The listing builds one solid part. Answer for the finished solid, in the listing's coordinates (mm). Face numbers are marked on the shaded views. A direction names the side the tool comes from. Round coordinates to 2 decimals unless told otherwise and drop trailing zeros. Loops run counter-clockwise (first coordinate to the right, second up) from the corner with the lowest first, then second, coordinate; pieces in that order, holes last. Notation, with made-up numbers: (-36, -11.5) - (-19, -11.5) arc R17 cw to (-19, 5.5) - close; hole circle Ø5 at (79.5, -12.75). An arc over 180 degrees is marked (long way). Write item = value, one per line. Start each with the question number.
1) Section A-A, the plane y = -25.5 is taken. Determine the outline of the cut face in (x, z), and give its area (3 significant figures).
2) Straight lines are drawn through the part: line 1 along Y through (x, z) = (55, 8.75); line 2 along X through (y, z) = (-25, 6); line 3 along X through (y, z) = (-6, 7.5). For each, find the intervals that lie inside material, in ascending order.
3) Section C-C, the plane x = 55 is taken. Determine the outline of the cut face in (y, z).
4) Section B-B, the plane z = 8.75 is taken. Determine the outline of the cut face in (x, y).
5) Section D-D, the plane z = 3.25 is taken. Determine the outline of the cut face in (x, y).
6) For a pull along X with two mould halves and no side action, classify the marked faces 1, 2 and 3 as released by +X, released by -X, zero draft, split by the parting line, or undercut.
7) A tool of negligible diameter and unlimited length cuts with its end or side. For the marked faces 4, 5, 6, 7 and 8, from which of +Z, -Z, +X, -X, +Y, -Y can it reach the whole face along a straight path? Write none if from no direction.
8) Given pin 1 Ø5 at (y, z) = (-31.5, 6.5) entering from -X; pin 2 Ø1.5 at (x, y) = (47.5, -11.5) entering from +Z; pin 3 Ø1.5 at (y, z) = (-21, 2.5) entering from +X; pin 4 Ø4 at (y, z) = (-24, 8.5) entering from +X, each flat-ended and moving along its own axis, determine where each tip first touches the part or whether it passes through.
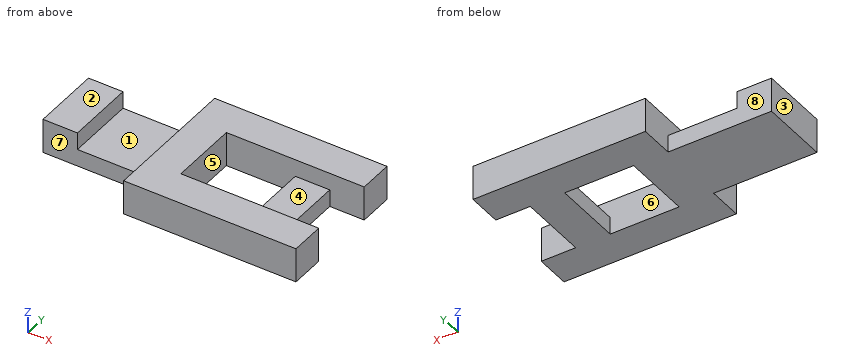
from build123d import *

# Parameters (mm, degrees)
F1_DEPTH  = 40
F3_DEPTH  = 10
F5_DEPTH  = 10
F6_W      = 10
F6_H      = 20
F7_DEPTH  = 25
F6_W_2    = 30
F8_DEPTH  = 5
F9_W      = 20
F9_H      = 20
F10_DEPTH = 25
F11_DEPTH = 10


with BuildPart() as f1:
    # F0 (on Front) → F1 (new body)
    with BuildSketch(Plane.XZ):
        Polygon((0, 10), (0, 0), (80, 0), (80, 10), (40, 10), (40, 5), (10, 5), (10, 10), align=None)
    extrude(amount=F1_DEPTH)

    # F2 (on face) → F3 (cut)
    with BuildSketch(Plane.XZ.offset(40)):
        Polygon((10, 10), (0, 10), (0, 0), (40, 0), (40, 5), (10, 5), align=None)
    extrude(amount=-F3_DEPTH, mode=Mode.SUBTRACT)

    # F4 (on face) → F5 (cut)
    with BuildSketch(Plane(origin=(0, 0, 0), x_dir=(-1, 0, 0), z_dir=(0, 1, 0))):
        Polygon((-40, 0), (0, 0), (0, 10), (-10, 10), (-10, 5), (-40, 5), align=None)
    extrude(amount=-F5_DEPTH, mode=Mode.SUBTRACT)

    # F6 (on face) → F7 (cut)
    with BuildSketch(Plane.XY.offset(10)):
        with Locations((75, -20)):
            Rectangle(F6_W, F6_H)
    extrude(amount=-F7_DEPTH, mode=Mode.SUBTRACT)

    # F6 (on face) → F8 (cut)
    with BuildSketch(Plane.XY.offset(10)):
        with Locations((55, -20)):
            Rectangle(F6_W_2, F6_H)
    extrude(amount=-F8_DEPTH, mode=Mode.SUBTRACT)

    # F9 (on face) → F10 (cut)
    with BuildSketch(Plane.XY.offset(10)):
        with Locations((50, -20)):
            Rectangle(F9_W, F9_H)
    extrude(amount=-F10_DEPTH, mode=Mode.SUBTRACT)

    # F9 (on face) → F11 (join)
    with BuildSketch(Plane.XY.offset(10)):
        Polygon((30, -40), (40, -40), (40, -30), (40, -10), (40, 0), (30, 0), align=None)
    extrude(amount=-F11_DEPTH)


solid = f1.part
Geometry check:
q1.outline = (0, 0) - (40, 0) - (40, 10) - (30, 10) - (30, 5) - (10, 5) - (10, 10) - (0, 10) - close; (60, 0) - (70, 0) - (70, 5) - (60, 5) - close
q1.area = 350 mm2
q2.line_1 = -40 to -30, -10 to 0
q2.line_2 = 0 to 10, 30 to 40
q2.line_3 = 30 to 80
q3.outline = (-40, 0) - (-30, 0) - (-30, 10) - (-40, 10) - close; (-10, 0) - (0, 0) - (0, 10) - (-10, 10) - close
q4.outline = (0, -30) - (10, -30) - (10, -10) - (0, -10) - close; (30, -40) - (80, -40) - (80, -30) - (40, -30) - (40, -10) - (80, -10) - (80, 0) - (30, 0) - close
q5.outline = (0, -30) - (30, -30) - (30, -40) - (80, -40) - (80, -30) - (70, -30) - (70, -10) - (80, -10) - (80, 0) - (30, 0) - (30, -10) - (0, -10) - close; hole (40, -30) - (60, -30) - (60, -10) - (40, -10) - close
q6.face_1 = undercut
q6.face_2 = zero draft
q6.face_3 = released by -X
q7.face_4 = +Z, +X
q7.face_5 = +Z, -Z
q7.face_6 = +Z
q7.face_7 = +Z, -Z, -X, -Y
q7.face_8 = +Z, -Z, -X, +Y
q8.pin_1 = 0
q8.pin_2 = through
q8.pin_3 = 70
q8.pin_4 = 40
